```python
from build123d import *

# Parameters (mm, degrees)
F1_DEPTH = 6.35


with BuildPart() as f1:
    # F0 (on Top) → F1 (new body)
    with BuildSketch(Plane.XY):
        Polygon((57.15, 130.81), (57.15, 152.4), (24.13, 152.4), (24.13, 146.05), (2.54, 146.05), (2.54, 152.4), (-16.51, 152.4), (-16.51, 146.05), (-38.1, 146.05), (-38.1, 152.4), (-57.15, 152.4), (-57.15, 130.81), (-63.5, 130.81), (-63.5, 111.76), (-57.15, 111.76), (-57.15, 90.17), (-63.5, 90.17), (-63.5, 71.12), (-57.15, 71.12), (-57.15, 49.53), (-63.5, 49.53), (-63.5, 30.48), (-57.15, 30.48), (-57.15, 8.89), (-63.5, 8.89), (-63.5, -10.16), (-57.15, -10.16), (-57.15, -31.75), (-63.5, -31.75), (-63.5, -50.8), (-57.15, -50.8), (-57.15, -72.39), (-63.5, -72.39), (-63.5, -91.44), (-57.15, -91.44), (-57.15, -113.03), (-63.5, -113.03), (-63.5, -132.08), (-57.15, -132.08), (-57.15, -152.4), (-38.1, -152.4), (-38.1, -146.05), (-16.51, -146.05), (-16.51, -152.4), (2.54, -152.4), (2.54, -146.05), (24.13, -146.05), (24.13, -152.4), (43.18, -152.4), (57.15, -152.4), (57.15, -132.08), (63.5, -132.08), (63.5, -113.03), (57.15, -113.03), (57.15, -91.44), (63.5, -91.44), (63.5, -72.39), (57.15, -72.39), (57.15, -50.8), (63.5, -50.8), (63.5, -31.75), (57.15, -31.75), (57.15, -10.16), (63.5, -10.16), (63.5, 8.89), (57.15, 8.89), (57.15, 30.48), (63.5, 30.48), (63.5, 49.53), (57.15, 49.53), (57.15, 71.12), (63.5, 71.12), (63.5, 90.17), (57.15, 90.17), (57.15, 111.76), (63.5, 111.76), (63.5, 130.81), align=None)
    extrude(amount=F1_DEPTH)


solid = f1.part
```
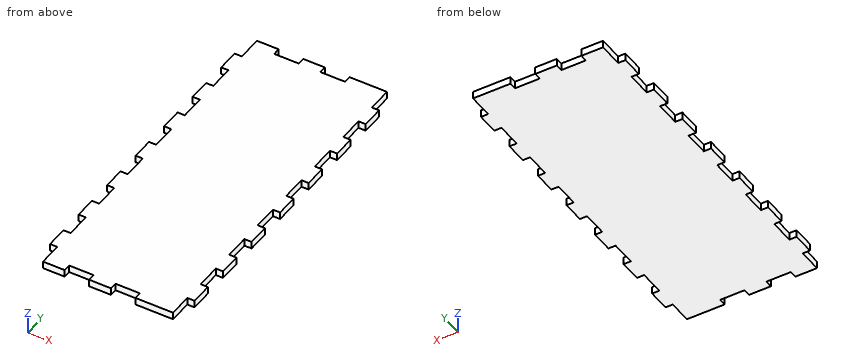
Design review of the part built by this model. Coordinates are the model's own, in mm. Coordinates: 2 decimals unless noted, no trailing zeros. Loops run counter-clockwise (first coordinate to the right, second up) from the corner with the lowest first, then second, coordinate; pieces in that order, holes last. Notation, with made-up numbers: M 13.25,44.25 L 48.25,44.25 A24 ccw 48.25,78.25 Z; hole C -2,-27.75 d1. An arc over 180 degrees is marked long. One line per question, with ' | ' between items.
(1) We need section B-B (x = -32.5). Give the boundary of the cut face in (y, z), and give its area (3 significant figures).
Filled in:
outline: M -146.05,0 L 146.05,0 L 146.05,6.35 L -146.05,6.35 Z | area: 1,850 mm^2
(2) For pin 1 Ø1.9 at (x, z) = (-61, 1.5) entering from +Y; pin 2 Ø3 at (y, z) = (-64, 3.5) entering from -X; pin 3 Ø1.9 at (y, z) = (-103.5, 3.5) entering from +X, all flat-tipped, find the tip position at first contact; note any pin that passes through.
Filled in:
pin 1: stops at y = 130.81 | pin 2: stops at x = -57.15 | pin 3: stops at x = 57.15
(3) We need section A-A (y = 102). Give the boundary of the cut face in (x, z), and give its area (3 significant figures).
Filled in:
outline: M -57.15,0 L 57.15,0 L 57.15,6.35 L -57.15,6.35 Z | area: 726 mm^2
(4) Wall thickness on probe 1 along Y at (x, z) = (-26, 4.5); probe 2 along X at (y, z) = (-19, 3.75): over which ranges is each line inside the solid? List them lowest first.
Filled in:
probe 1: y = -146.05 to 146.05 | probe 2: x = -57.15 to 57.15
